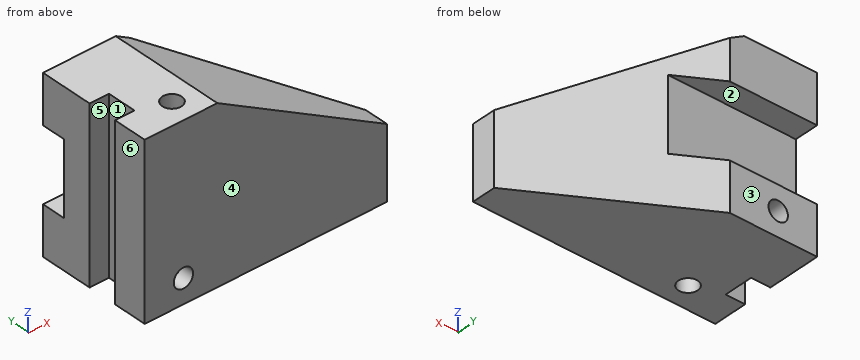
```python
from build123d import *

# Parameters (mm, degrees)
EXTRUDE_3_DEPTH     = 175
CUT_EXTRUDE_2_DEPTH = 220
SKETCH_9_W          = 75
SKETCH_9_H          = 25
CUT_EXTRUDE_3_DEPTH = 220
SKETCH_10_W         = 20
SKETCH_10_H         = 30
CUT_EXTRUDE_4_DEPTH = 220
SKETCH_11_R         = 10
CUT_EXTRUDE_5_DEPTH = 220
SKETCH_12_R         = 10
CUT_EXTRUDE_6_DEPTH = 220


with BuildPart() as part:
    # 草图7 → 凸台-拉伸3 (new body)
    with BuildSketch(Plane.XY):
        Polygon((0, 0), (250, 0), (250, 25), (90, 120), (0, 120), align=None)
    extrude(amount=EXTRUDE_3_DEPTH)

    # 草图8 → 切除-拉伸2 (cut)
    with BuildSketch(Plane(origin=(0, 0, 0), x_dir=(1, 0, 0), z_dir=(0, 1, 0))):
        Polygon((75, -175), (250, -73.963702892), (250, -175), align=None)
    extrude(amount=CUT_EXTRUDE_2_DEPTH, mode=Mode.SUBTRACT)

    # 草图9 → 切除-拉伸3 (cut)
    with BuildSketch(Plane.ZY):
        with Locations((87.5, 107.5)):
            Rectangle(SKETCH_9_W, SKETCH_9_H)
    extrude(amount=-CUT_EXTRUDE_3_DEPTH, mode=Mode.SUBTRACT)

    # 草图10 → 切除-拉伸4 (cut)
    with BuildSketch(Plane.XY.offset(175)):
        with Locations((10, 50)):
            Rectangle(SKETCH_10_W, SKETCH_10_H)
    extrude(amount=-CUT_EXTRUDE_4_DEPTH, mode=Mode.SUBTRACT)

    # 草图11 → 切除-拉伸5 (cut)
    with BuildSketch(Plane.XY.offset(175)):
        with Locations((50, 25)):
            Circle(SKETCH_11_R)
    extrude(amount=-CUT_EXTRUDE_5_DEPTH, mode=Mode.SUBTRACT)

    # 草图12 → 切除-拉伸6 (cut)
    with BuildSketch(Plane(origin=(0, 120, 0), x_dir=(1, 0, 0), z_dir=(0, 1, 0))):
        with Locations(Location((40, -25, 0), (0, 0, 180))):
            Circle(SKETCH_12_R)
    extrude(amount=-CUT_EXTRUDE_6_DEPTH, mode=Mode.SUBTRACT)


solid = part.part
```
Design review of the part built by this model. Coordinates are the model's own, in mm. Face numbers are marked on the shaded views. A direction names the side the tool comes from. Give positions to 0.01 mm unless a question says otherwise; leave off trailing zeros. Write each loop counter-clockwise with the first axis right and the second up, starting at its lowest first coordinate (ties: lowest second). Pieces come first, ordered by that corner, then holes.
(1) Add section D-D (x = 70.5). Give the boundary of the cut face in (y, z), and give its area (3 significant figures).
Checked values:
outline: (0, 0) - (120, 0) - (120, 50) - (95, 50) - (95, 125) - (120, 125) - (120, 175) - (0, 175) - close
area: 19,100 mm2
(2) Add section A-A (z = 25). Give the boundary of the cut face in (x, y), and give its area (3 significant figures).
Checked values:
outline: (0, 0) - (30, 0) - (30, 120) - (0, 120) - (0, 65) - (20, 65) - (20, 35) - (0, 35) - close; (50, 0) - (250, 0) - (250, 25) - (90, 120) - (50, 120) - (50, 35) arc R10 cw to (50, 15) - close
area: 19,200 mm2
(3) Wall thickness on line 1 along Z through (x, y) = (40, 44); line 2 along Y through (x, z) = (50, 133); line 3 along X through (y, z) = (25, 58): over which ranges is each line inside the solid? List them lowest first.
Checked values:
line 1: z = 0 to 15, 35 to 175
line 2: y = 0 to 15, 35 to 120
line 3: x = 0 to 40, 60 to 250
(4) Clearance check with flat-ended pins moving along their axes: pin 1 Ø8 at (y, z) = (65, 79.5) entering from +X; pin 2 Ø9 at (y, z) = (54.5, 113.5) entering from -X; pin 3 Ø12.5 at (x, y) = (55.5, 106) entering from -Z; pin 4 Ø18 at (x, z) = (40, 25) entering from +Y. State where each tip first meets the part, or that it passes through.
Checked values:
pin 1: stops at x = 189.37
pin 2: stops at x = 20
pin 3: stops at z = 0
pin 4: passes through
(5) Add section C-C (z = 64.5). Give the boundary of the cut face in (x, y), and give its area (3 significant figures).
Checked values:
outline: (0, 0) - (250, 0) - (250, 25) - (132.11, 95) - (0, 95) - (0, 65) - (20, 65) - (20, 35) - (0, 35) - close; hole circle Ø20 at (50, 25)
area: 18,700 mm2
(6) Tool access review of the marked faces 1, 2 and 3: name each direction out of +Z, -Z, +X, -X, +Y, -Y from which nothing blocks a thin tool from reaching the whole face with its end or side.
Checked values:
face 1: +Z, -Z, -X
face 2: +X, -X, +Y
face 3: +Z, -Z, +X, -X, +Y
(7) Mouldability with a two-part tool opening along Y and no side actions: class the marked faces 4, 5 and 6 as +Y half, -Y half, draft (parallel to the pull), parting line (faces both ways), or undercut.
Checked values:
face 4: -Y half
face 5: undercut
face 6: draft
(8) Add section B-B (y = 101). Give the boundary of the cut face in (x, z).
Checked values:
outline: (0, 0) - (122, 0) - (122, 50) - (0, 50) - close; (0, 125) - (122, 125) - (122, 147.86) - (75, 175) - (0, 175) - close; hole circle Ø20 at (40, 25)
